Autodesk Inventor part; units mm, degrees
ref_plane "YZ Plane" through (0, 0, 0) normal (1, 0, 0) x (0, 1, 0)
ref_plane "XZ Plane" through (0, 0, 0) normal (0, 1, 0) x (-1, 0, 0)
ref_plane "XY Plane" through (0, 0, 0) normal (0, 0, 1) x (1, 0, 0)
sketch "Sketch1" plane through (0, 0, 0) normal (0, 0, 1) x (1, 0, 0)
  line L0 (203.2, 196.85) -> (-203.2, 196.85)
  line L1 (-203.2, 196.85) -> (-203.2, -196.85)
  line L2 (-203.2, -196.85) -> (203.2, -196.85)
  line L3 (203.2, -196.85) -> (203.2, 196.85)
  point P0 (0, 0)
  dimension "d0" = 393.7
  dimension "d1" = 406.4
  dimension "d2" = 203.2
  dimension "d3" = 196.85
extrude "Extrusion1" add sketch "Sketch1" along normal mid plane 3.175
sketch "Sketch2" plane through (0, 0, 1.5875) normal (0, 0, 1) x (1, 0, 0)
  circle A0 centre (-6.35, 0) radius 31.75
  point P0 (0, 0)
  dimension "d6" = 63.5
  dimension "d20" = 6.35
extrude "Extrusion2" cut sketch "Sketch2" against normal through all
fillet "Fillet1" radius 3.175 4 edges at (203.2, -196.85, 0) (-203.2, -196.85, 0) (-203.2, 196.85, 0) (203.2, 196.85, 0)
sketch "Sketch3" plane through (0, 0, 1.5875) normal (0, 0, 1) x (1, 0, 0)
  line L0 (138.5, 173.4) -> (131.9, 173.4)
  line L1 (131.9, 173.4) -> (131.9, 163.8)
  line L2 (131.9, 163.8) -> (138.5, 163.8)
  line L3 (138.5, 163.8) -> (138.5, 173.4)
  line L4 (135.2, 173.4) -> (135.2, 163.8) construction
  line L5 (203.2, -193.675) -> (203.2, 193.675)
  line L6 (200.025, 196.85) -> (-200.025, 196.85)
  line L7 (138.5, 168.6) -> (131.9, 168.6) construction
  point P0 (0, 0)
  dimension "d11" = 6.6
  dimension "d12" = 68
  dimension "d14" = 9.6
  dimension "d18" = 28.25
extrude "Extrusion3" cut sketch "Sketch3" against normal through all
fillet "Fillet2" radius 3.3 4 edges at (138.5, 173.4, 0) (131.9, 173.4, 0) (138.5, 163.8, 0) (131.9, 163.8, 0)
mirror "Mirror1" about plane through (0, 0, 0) normal (0, 1, 0) of "Extrusion3", "Fillet2"
mirror "Mirror2" about plane through (0, 0, 0) normal (1, 0, 0) of "Extrusion3", "Fillet2", "Mirror1"
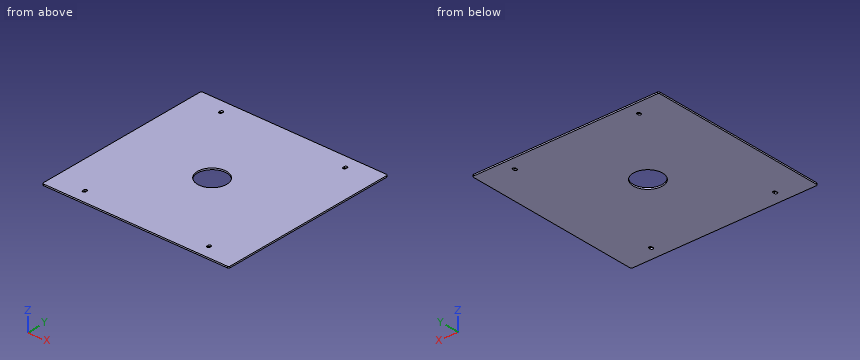
The model under review builds one solid part; all positions refer to its coordinate system, in mm. Coordinates: 2 decimals unless noted, no trailing zeros. Write each loop counter-clockwise with the first axis right and the second up, starting at its lowest first coordinate (ties: lowest second). Pieces come first, ordered by that corner, then holes. Notation, with made-up numbers: (22, -17) -> (31, -17) arc R27 cw to (31, 4) -> close; hole circle Ø9 at (17.25, -3). An arc over 180 degrees is marked (long way). One line per item, written item: value. Start each with the question number.
Q1. To check wall thickness, follow probe 1 along Y at (x, z) = (-6.35, -0.45); probe 2 along X at (y, z) = (-18, -0.1); probe 3 along Y at (x, z) = (20.5, -0.4). State the ranges of each line that lie inside material, in increasing order.
Q2. Add section B-B, the plane y = 0. Give the boundary of the cut face in (x, z).
Q3. Add section A-A, the plane x = -6.35. Give the boundary of the cut face in (y, z), then the cut area to 3 significant figures.
Response:
1. probe 1: -196.85 to -31.75, 31.75 to 196.85
1. probe 2: -203.2 to -32.5, 19.8 to 203.2
1. probe 3: -196.85 to -16.95, 16.95 to 196.85
2. outline: (-203.2, -1.59) -> (-38.1, -1.59) -> (-38.1, 1.59) -> (-203.2, 1.59) -> close; (25.4, -1.59) -> (203.2, -1.59) -> (203.2, 1.59) -> (25.4, 1.59) -> close
3. outline: (-196.85, -1.59) -> (-31.75, -1.59) -> (-31.75, 1.59) -> (-196.85, 1.59) -> close; (31.75, -1.59) -> (196.85, -1.59) -> (196.85, 1.59) -> (31.75, 1.59) -> close
3. area: 1,050 mm²
